Here's the drawing with two shaded views (mm, measured from the low corner). I have some questions. Round coordinates to 2 decimals unless told otherwise and drop trailing zeros. Loops run counter-clockwise (first coordinate to the right, second up) from the corner with the lowest first, then second, coordinate; pieces in that order, holes last. Notation, with made-up numbers: (50, 40.5) - (106, 40.5) arc R29 ccw to (106, 72.5) - close; hole circle Ø1 at (62, 47). An arc over 180 degrees is marked (long way). Use one line per item in the form item = value.
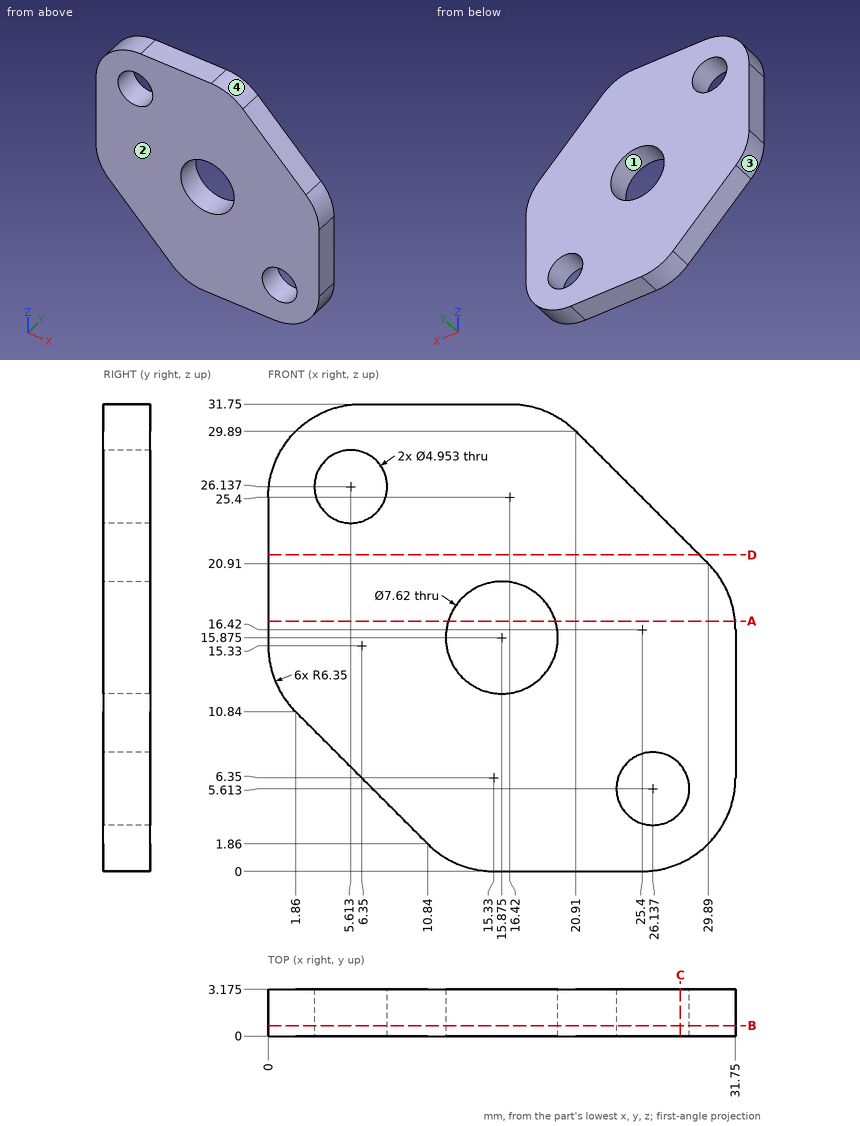
1. If we section it at D-D, the plane z = 21.5: Write out the boundary of the cut face in (x, y) (1 decimal).
Solution:
outline = (0, 0) - (29.3, 0) - (29.3, 3.2) - (0, 3.2) - close
2. Please list where these lines run through material, in increasing order: line 1 along Z through (x, y) = (16, 0.9); line 2 along Z through (x, y) = (24.5, 0.4) (1 decimal).
Solution:
line_1 = 0 to 12.07, 19.68 to 31.75
line_2 = 0 to 3.8, 7.5 to 26.3
3. We'd pull the mould along X, two halves only. Please class the marked faces 1, 2, 3 and 4: +X half, -X half, draft (parallel to the pull), parting line (faces both ways), or undercut.
Solution:
face_1 = undercut
face_2 = draft
face_3 = -X half
face_4 = +X half
4. If we section it at A-A, the plane z = 17: Write out the boundary of the cut face in (x, y) (1 decimal), plus the area to 3 significant figures.
Solution:
outline = (0, 0) - (12.2, 0) - (12.2, 3.2) - (0, 3.2) - close; (19.5, 0) - (31.7, 0) - (31.7, 3.2) - (19.5, 3.2) - close
area = 77.6 mm^2
5. For P1, Ø3, axis at x = 26.14, z = 5.61, coming from the +Y side, with a flat end and sliding along its axis, tell me the tip position at first contact or that it passes through.
Solution:
P1 = through
6. If we section it at C-C, the plane x = 28: Write out the boundary of the cut face in (y, z) (1 decimal).
Solution:
outline = (0, 0.6) - (3.2, 0.6) - (3.2, 4) - (0, 4) - close; (0, 7.2) - (3.2, 7.2) - (3.2, 22.8) - (0, 22.8) - close
7. If we section it at B-B, the plane y = 0.7: Count the separate pieces of the cut face and the enclosed holes in it, plus the area to 3 significant figures.
Solution:
separate_pieces = 1
enclosed_holes = 3
area = 742 mm^2
